Autodesk Inventor part; units mm, degrees
ref_plane "YZ Plane" through (0, 0, 0) normal (1, 0, 0) x (0, 1, 0)
ref_plane "XZ Plane" through (0, 0, 0) normal (0, 1, 0) x (-1, 0, 0)
ref_plane "XY Plane" through (0, 0, 0) normal (0, 0, 1) x (1, 0, 0)
sketch "Sketch1" plane through (0, 0, 0) normal (0, 1, 0) x (-1, 0, 0)
  circle A0 centre (0, 0) radius 4
  dimension "d0" = 8
extrude "Extrusion1" add sketch "Sketch1" along normal blind 7
sketch "Sketch2" plane through (0, 7, 0) normal (0, 1, 0) x (1, 0, 0)
  circle A0 centre (0, 0) radius 5.75
  dimension "d3" = 11.5
extrude "Extrusion2" add sketch "Sketch2" along normal blind 3.2
sketch "Sketch4" plane through (0, 0, 0) normal (1, 0, 0) x (0, 1, 0)
  line L0 (20.4, 3.1121) -> (19.5121, 4)
  line L1 (19.5121, 4) -> (17.7879, 4)
  line L2 (16.9, 3.1121) -> (17.7879, 4)
  line L3 (13.4, 3.1121) -> (14.2879, 4)
  line L4 (14.2879, 4) -> (16.0121, 4)
  line L5 (16.9, 3.1121) -> (16.0121, 4)
  line L6 (13.4, 3.1121) -> (13.4, 6.6121)
  line L7 (13.4, 8.5445) -> (20.4, 8.5445)
  line L8 (20.4, 8.5445) -> (20.4, 3.1121)
  line L9 (0, 3.1121) -> (0.8879, 4)
  line L10 (0.8879, 4) -> (2.6121, 4)
  line L11 (3.5, 3.1121) -> (2.6121, 4)
  line L12 (3.5, 3.1121) -> (4.3879, 4)
  line L13 (6.1121, 4) -> (4.3879, 4)
  line L14 (7, 3.1121) -> (6.1121, 4)
  line L15 (7, 3.1121) -> (7, 6.6121)
  line L16 (7, 8.5445) -> (0, 8.5445)
  line L17 (0, 8.5445) -> (0, 3.1121)
  line L18 (13.4, 6.6121) -> (7, 6.6121)
  line L19 (13.4, 8.5445) -> (7, 8.5445)
  line L20 (-4.08, 0) -> (24.48, 0)
  point P0 (0, 0)
revolve "Revolution1" cut sketch "Sketch4" angle 360 about axis through (0, -10, 0) along (0, 1, 0)
hole "Hole2" at (0, 0, 0) direction (0, 1, 0) diameter 4.4 end through all
properties part number "Split spacer"
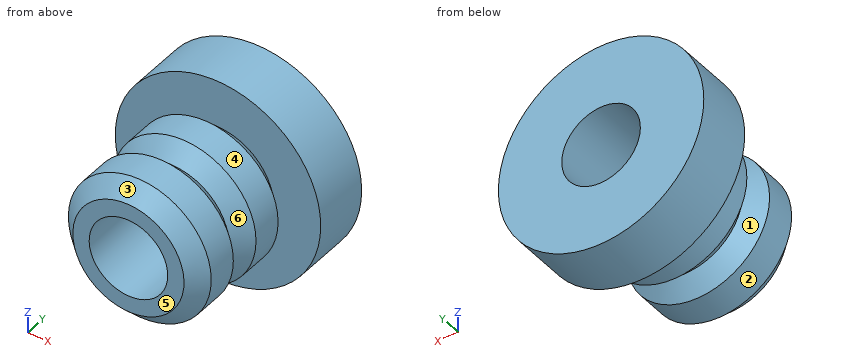
For this review, take the finished solid that the model builds, in its own axes (mm). Face numbers are marked on the shaded views. A direction names the side the tool comes from. Coordinates: 2 decimals unless noted, no trailing zeros. Loops run counter-clockwise (first coordinate to the right, second up) from the corner with the lowest first, then second, coordinate; pieces in that order, holes last.
1. For the marked faces 4, 5 and 6, list the 3-axis set-ups (+Z, -Z, +X, -X, +Y, -Y) from which the entire face can be reached by the end or side of a thin tool; tool diameter is ignored.
2. Insertion check: P1, Ø5, axis at y = 6.5, z = 3, coming from the +X side; P2, Ø3, axis at x = -4, z = 4.5, coming from the -Y side; P3, Ø1.5, axis at x = 1.5, y = 4, coming from the +Z side; P4, Ø4, axis at x = 0, z = 0, coming from the +Y side. Each pin has a flat end and moves straight along its axis. Give the tip position at first contact, or say it passes through.
3. Add section D-D, the plane y = 8.5. Give the boundary of the cut face in (x, z), then the cut area to 3 significant figures.
4. Add section B-B, the plane x = 0. Give the boundary of the cut face in (y, z).
5. Add section C-C, the plane y = 2.25. Give the boundary of the cut face in (x, z), then the cut area to 3 significant figures.
6. Add section A-A, the plane z = 0. Give the boundary of the cut face in (x, y).
7. For line 1 (Z direction, x = 0, y = 5.75); line 2 (Z direction, x = 0, y = 7.25), list the stretches that pass through material, from the lowest coordinate up.
8. Mouldability with a two-part tool opening along Y and no side actions: class the marked faces 1, 2 and 3 as +Y half, -Y half, draft (parallel to the pull), parting line (faces both ways), or undercut.
Result:
1. face 4: -Y
1. face 5: +Z, -Z, +X, -X, -Y
1. face 6: none
2. P1: stops at x = 5.72
2. P2: stops at y = 7
2. P3: stops at z = 3.91
2. P4: passes through
3. outline: circle Ø11.5 at (0, 0); hole circle Ø4.4 at (0, 0)
3. area: 88.7 mm2
4. outline: (0, -3.11) - (0.89, -4) - (2.61, -4) - (3.5, -3.11) - (4.39, -4) - (6.11, -4) - (7, -3.11) - (7, -5.75) - (10.2, -5.75) - (10.2, -2.2) - (0, -2.2) - close; (0, 2.2) - (10.2, 2.2) - (10.2, 5.75) - (7, 5.75) - (7, 3.11) - (6.11, 4) - (4.39, 4) - (3.5, 3.11) - (2.61, 4) - (0.89, 4) - (0, 3.11) - close
5. outline: circle Ø8 at (0, 0); hole circle Ø4.4 at (0, 0)
5. area: 35.1 mm2
6. outline: (-5.75, 7) - (-3.11, 7) - (-4, 6.11) - (-4, 4.39) - (-3.11, 3.5) - (-4, 2.61) - (-4, 0.89) - (-3.11, 0) - (-2.2, 0) - (-2.2, 10.2) - (-5.75, 10.2) - close; (2.2, 0) - (3.11, 0) - (4, 0.89) - (4, 2.61) - (3.11, 3.5) - (4, 4.39) - (4, 6.11) - (3.11, 7) - (5.75, 7) - (5.75, 10.2) - (2.2, 10.2) - close
7. line 1: z = -4 to -2.2, 2.2 to 4
7. line 2: z = -5.75 to -2.2, 2.2 to 5.75
8. face 1: undercut
8. face 2: draft
8. face 3: -Y half
